from build123d import *

# Parameters (mm, degrees)
SKETCH1_W           = 15.8
SKETCH1_H           = 15.8
SKETCH1_W_2         = 13.8
SKETCH1_H_2         = 13.8
BOSS_EXTRUDE2_DEPTH = 500
SKETCH4_R           = 2.25
CUT_EXTRUDE2_DEPTH  = 501.311952686
SKETCH6_R           = 2.25
CUT_EXTRUDE3_DEPTH  = 501.311952686


with BuildPart() as part:
    # Sketch1 → Boss-Extrude2 (new body)
    with BuildSketch(Plane(origin=(0, 0, 0), x_dir=(1, 0, 0), z_dir=(0, 1, 0))):
        Rectangle(SKETCH1_W, SKETCH1_H)
        Rectangle(SKETCH1_W_2, SKETCH1_H_2, mode=Mode.SUBTRACT)
    extrude(amount=BOSS_EXTRUDE2_DEPTH)

    # Sketch4 → Cut-Extrude2 (cut, through all)
    with BuildSketch(Plane(origin=(0, 0, -7.9), x_dir=(-1, 0, 0), z_dir=(0, 0, -1))):
        with Locations(Location((-0.094266251, 438, 0), (0, 0, 180))):
            Circle(SKETCH4_R)
        with Locations((-0.094266251, 62)):
            Circle(SKETCH4_R)
    extrude(amount=-CUT_EXTRUDE2_DEPTH, mode=Mode.SUBTRACT)

    # Sketch6 → Cut-Extrude3 (cut, through all)
    with BuildSketch(Plane(origin=(7.9, 0, 0), x_dir=(0, 0, -1), z_dir=(1, 0, 0))):
        with Locations((0, 262)):
            Circle(SKETCH6_R)
        with Locations((0, 238)):
            Circle(SKETCH6_R)
    extrude(amount=-CUT_EXTRUDE3_DEPTH, mode=Mode.SUBTRACT)


solid = part.part
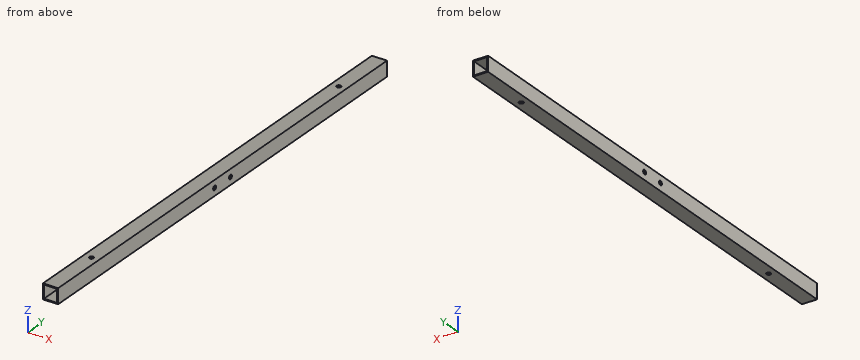
For this review, take the finished solid that the model builds, in its own axes (mm). Round coordinates to 2 decimals unless told otherwise and drop trailing zeros. Loops run counter-clockwise (first coordinate to the right, second up) from the corner with the lowest first, then second, coordinate; pieces in that order, holes last. Notation, with made-up numbers: (43.25, -28) - (85.25, -28) arc R22 ccw to (85.25, 10) - close; hole circle Ø4 at (54, 77). An arc over 180 degrees is marked (long way). Use one line per item in the form item = value.
Item 1: Consider section A-A on y = 70. Write out the cut boundary in (x, z), then the cut area to 3 significant figures.
Answers:
outline = (-7.9, -7.9) - (7.9, -7.9) - (7.9, 7.9) - (-7.9, 7.9) - close; hole (-6.9, -6.9) - (6.9, -6.9) - (6.9, 6.9) - (-6.9, 6.9) - close
area = 59.2 mm^2
Item 2: For line 1 (Y direction, x = 7.25, z = 0); line 2 (Z direction, x = -2, y = 264.5); line 3 (Z direction, x = 7.35, y = 238), list the stretches that pass through material, from the lowest coordinate up.
Answers:
line_1 = 0 to 235.75, 240.25 to 259.75, 264.25 to 500
line_2 = -7.9 to -6.9, 6.9 to 7.9
line_3 = -7.9 to -2.25, 2.25 to 7.9
Item 3: Clearance check with a flat-ended pin moving along its axis: P1, Ø4, axis at y = 238, z = 0, coming from the -X side. State where the tip first meets the part, or that it passes through.
Answers:
P1 = through
